Could you check a few things on this drawing? It's one solid part, dimensions in mm from its lowest x, y, z. Give positions to 0.01 mm unless a question says otherwise; leave off trailing zeros. Write each loop counter-clockwise with the first axis right and the second up, starting at its lowest first coordinate (ties: lowest second). Pieces come first, ordered by that corner, then holes. Notation, with made-up numbers: (73, 57) -> (128, 57) arc R13 ccw to (128, 66) -> close; hole circle Ø11 at (86, 36.25). An arc over 180 degrees is marked (long way). Use CSV: the item, a comma, the result in double quotes. Start each with the question number.
(1) Suppose I cut it at B-B on x = 52. List the corners of the cut face in (y, z) for me.
(2) For pin 1 Ø0.5 at (x, z) = (37, 0.5) entering from -Y (3 decimals); pin 2 Ø0.5 at (y, z) = (1, 1) entering from -X; pin 3 Ø0.8 at (x, z) = (47, 0.5) entering from -Y, each with a flat end and sliding along its axis, tell me the tip position at first contact or that it passes through.
(3) Suppose I cut it at A-A on z = 1.1. List the corners of the cut face in (x, y) for me (3 decimals), plus the area to 3 significant figures.
(4) I need wall thicknesses on L1, parallel to X at y = 1.25, z = 0.1; L2, parallel to X at y = 2.25, z = 1.55; L3, parallel to X at y = 10, z = 0.1. Which ranges of each line are inside material? Lowest first, please. Write a range as [from, to].
(5) Suppose I cut it at C-C on y = 8.25. List the corners of the cut face in (x, z) for me.
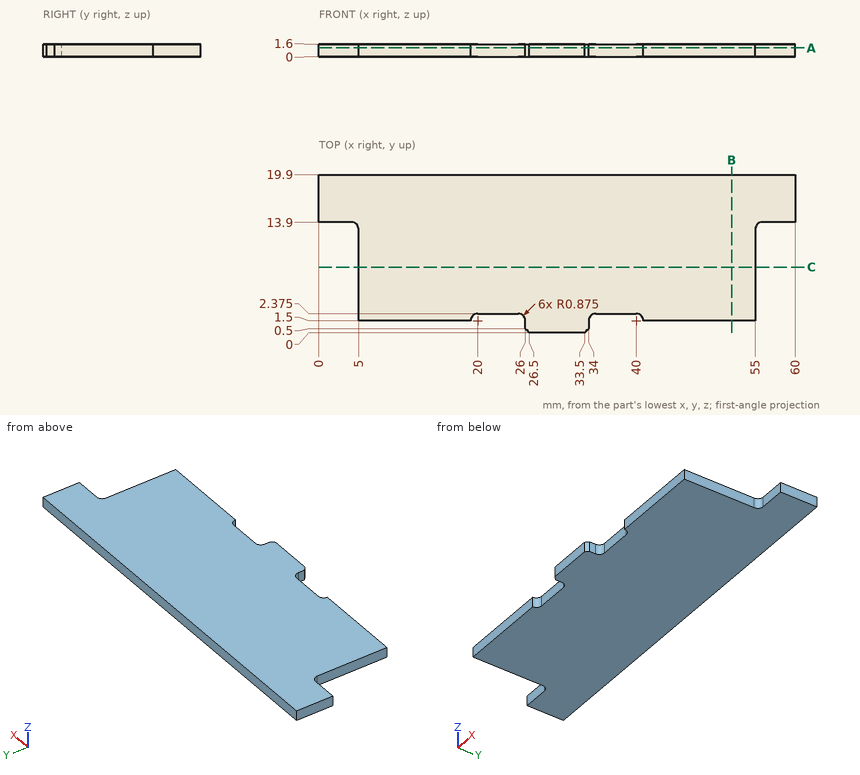
Geometry says:
1,outline,"(1.5, 0) -> (19.9, 0) -> (19.9, 1.6) -> (1.5, 1.6) -> close"
2,pin 1,"y = 2.375"
2,pin 2,"x = 26"
2,pin 3,"y = 1.5"
3,outline,"(0, 13.9) -> (4.125, 13.9) arc R0.875 cw to (5, 13.025) -> (5, 1.5) -> (19.125, 1.5) arc R0.875 cw to (20, 2.375) -> (25.125, 2.375) arc R0.875 cw to (26, 1.5) -> (26, 0.5) -> (26.5, 0) -> (33.5, 0) -> (34, 0.5) -> (34, 1.5) arc R0.875 cw to (34.875, 2.375) -> (40, 2.375) arc R0.875 cw to (40.875, 1.5) -> (55, 1.5) -> (55, 13.025) arc R0.875 cw to (55.875, 13.9) -> (60, 13.9) -> (60, 19.9) -> (0, 19.9) -> close"
3,area,"981 mm²"
4,L1,"[26, 34]"
4,L2,"[5, 19.55], [25.58, 34.42], [40.45, 55]"
4,L3,"[5, 55]"
5,outline,"(5, 0) -> (55, 0) -> (55, 1.6) -> (5, 1.6) -> close"
